```python
from build123d import *

# Parameters (mm, degrees)
F0_W        = 127
F0_H        = 76.2
F0_R        = 5.7659781113
F0_R_2      = 12.8582731401
F0_R_3      = 5.2319601114
F0_R_4      = 13.6233305285
F0_R_5      = 5.1796195503
F0_R_6      = 10.9267536549
F0_R_7      = 8.7936415442
F0_R_8      = 6.5428428961
F0_R_9      = 6.35
F1_DEPTH    = 50.8
F2_R        = 7.4007288491
F3_DEPTH    = 51.054
F4_T1_DEPTH = 153.1282991577
F5_R        = 5.08


# Not quite as in the source:
# - a fillet or chamfer that OpenCascade refuses, or shapes differently, is made with other operations: its cross-section is extruded or revolved along the edge and cut away or added


with BuildPart() as f1:
    # F0 (on Front) → F1 (new body)
    with BuildSketch(Plane.XZ):
        with Locations((1.9998494536, 3.723031328)):
            Rectangle(F0_W, F0_H)
        with Locations((-50.9259700775, -19.3260908127)):
            Circle(F0_R, mode=Mode.SUBTRACT)
        with Locations((-24.3451949209, -17.612459138)):
            Circle(F0_R_2, mode=Mode.SUBTRACT)
        with Locations((7.3802489787, -12.4715631828)):
            Circle(F0_R_3, mode=Mode.SUBTRACT)
        with Locations((38.248244673, -14.6136032417)):
            Circle(F0_R_4, mode=Mode.SUBTRACT)
        with Locations((-35.9206944704, 4.664753098)):
            Circle(F0_R_5, mode=Mode.SUBTRACT)
        with Locations((-5.4814172909, 21.3726628572)):
            Circle(F0_R_6, mode=Mode.SUBTRACT)
        with Locations((-43.6376929283, 28.6555960774)):
            Circle(F0_R_7, mode=Mode.SUBTRACT)
        with Locations((23.2429709285, 6.3783847727)):
            Circle(F0_R_8, mode=Mode.SUBTRACT)
        with Locations((46.4498494536, 16.423031328)):
            Circle(F0_R_9, mode=Mode.SUBTRACT)
    extrude(amount=F1_DEPTH)

    # F2 (on face) → F3 (cut)
    with BuildSketch(Plane.XZ.offset(50.8)):
        with Locations((21.7594634742, 25.6567392498)):
            Circle(F2_R)
    extrude(amount=-F3_DEPTH, mode=Mode.SUBTRACT)

    # F4: chamfer of 5.08 on 1 edges, made by hand

    # F4_s2 → F4_t1 (cut)
    with BuildSketch(Plane.YZ.offset(-74.5643001253)):
        Polygon((-45.72, 41.823031328), (-50.8, 36.743031328), (-50.8, 41.823031328), align=None)
    extrude(amount=F4_T1_DEPTH, mode=Mode.SUBTRACT)

    # F5
    f5_edges = [f1.edges().sort_by_distance(p)[0] for p in [
        (-61.500151, -22.86, 41.823031),
    ]]
    fillet(f5_edges, radius=F5_R)


solid = f1.part
```
Design review of the part built by this model. Coordinates are the model's own, in mm. Coordinates: 2 decimals unless noted, no trailing zeros. Loops run counter-clockwise (first coordinate to the right, second up) from the corner with the lowest first, then second, coordinate; pieces in that order, holes last. Notation, with made-up numbers: (-28, -1.75) -> (8, -1.75) arc R11 cw to (8, 18.25) -> close; hole circle Ø5 at (39, -18). An arc over 180 degrees is marked (long way). Answer as a JSON object with one key per item and string values.
Q1. Take a section at B-B on y = -39.5. Give the number of separate pieces and of enclosed holes in the cut face, plus the area to 3 significant figures.
Answer block:
{"separate pieces": "1", "enclosed holes": "10", "area": "7,240 mm^2"}
Q2. Take a section at A-A on x = 33. Give the boundary of the cut face in (y, z).
Answer block:
{"outline": "(-50.8, -34.38) -> (0, -34.38) -> (0, -27.19) -> (-50.8, -27.19) -> close; (-50.8, -2.04) -> (0, -2.04) -> (0, 41.82) -> (-45.72, 41.82) -> (-50.8, 36.74) -> close"}
Q3. To check wall thickness, follow L1, parallel to X at y = -40.5, z = 22; L2, parallel to X at y = -33.5, z = 8; L3, parallel to Z at x = -33.5, y = -36. State the ranges of each line that lie inside material, in increasing order.
Answer block:
{"L1": "x = -61.5 to -49.38, -37.89 to -16.39, 5.43 to 15.33, 28.19 to 43.41, 49.49 to 65.5", "L2": "x = -61.5 to -39.88, -31.96 to 16.9, 29.58 to 65.5", "L3": "z = -34.38 to -26.64, -8.58 to 0.09, 9.24 to 41.82"}
Q4. The part is to be moulded in two halves that separate along Z. For faces 1 (the flat face through (65.5, -25, 3)), 2 (the flat face through (4, -23, 41.823)), 3 (the cylindrical face through (16.706, -25.044, 6.666)), say which applies: +Z half, -Z half, draft (parallel to the pull), parting line (faces both ways), or undercut.
Answer block:
{"face 1": "draft", "face 2": "+Z half", "face 3": "undercut"}
Q5. Take a section at D-D on x = -20.5. Give the boundary of the cut face in (y, z).
Answer block:
{"outline": "(-50.8, -34.38) -> (0, -34.38) -> (0, -29.88) -> (-50.8, -29.88) -> close; (-50.8, -5.34) -> (0, -5.34) -> (0, 41.82) -> (-45.72, 41.82) -> (-50.8, 36.74) -> close"}
Q6. Take a section at C-C on x = -50. Give the boundary of the cut face in (y, z).
Answer block:
{"outline": "(-50.8, -34.38) -> (0, -34.38) -> (0, -25.02) -> (-50.8, -25.02) -> close; (-50.8, -13.63) -> (0, -13.63) -> (0, 22.59) -> (-50.8, 22.59) -> close; (-50.8, 34.73) -> (0, 34.73) -> (0, 41.82) -> (-45.72, 41.82) -> (-50.8, 36.74) -> close"}
